```python
from build123d import *

# Parameters (mm, degrees)
SKETCH1_R           = 5
SKETCH1_W           = 15
SKETCH1_H           = 110
BOSS_EXTRUDE1_DEPTH = 10
SKETCH1_3_W         = 15
SKETCH1_3_H         = 110
BOSS_EXTRUDE2_DEPTH = 20
SKETCH2_W           = 10
SKETCH2_H           = 30
CUT_EXTRUDE1_DEPTH  = 20


with BuildPart() as part:
    # Sketch1 → Boss-Extrude1 (new body)
    with BuildSketch(Plane.XY):
        with BuildLine():
            Line((70.181538652, 27.177394162), (-59.818461348, 27.177394162))
            ThreePointArc((-59.818461348, 27.177394162), (-114.818461348, -27.822605838), (-59.818461348, -82.822605838))
            Line((-59.818461348, -82.822605838), (70.181538652, -82.822605838))
            Line((70.181538652, -82.822605838), (70.181538652, 27.177394162))
        make_face()
        with Locations((-59.818461348, -27.822605838)):
            Circle(SKETCH1_R, mode=Mode.SUBTRACT)
        with Locations((77.681538652, -27.822605838)):
            Rectangle(SKETCH1_W, SKETCH1_H)
    extrude(amount=-BOSS_EXTRUDE1_DEPTH)

    # Sketch1_3 → Boss-Extrude2 (add)
    with BuildSketch(Plane.XY):
        with Locations((77.681538652, -27.822605838)):
            Rectangle(SKETCH1_3_W, SKETCH1_3_H)
    extrude(amount=BOSS_EXTRUDE2_DEPTH)

    # Sketch2 → Cut-Extrude1 (cut)
    with BuildSketch(Plane(origin=(85.181538652, 0, 0), x_dir=(0, 0, -1), z_dir=(1, 0, 0))):
        with Locations((-5, -27.822605838)):
            Rectangle(SKETCH2_W, SKETCH2_H)
    extrude(amount=-CUT_EXTRUDE1_DEPTH, mode=Mode.SUBTRACT)


solid = part.part
```
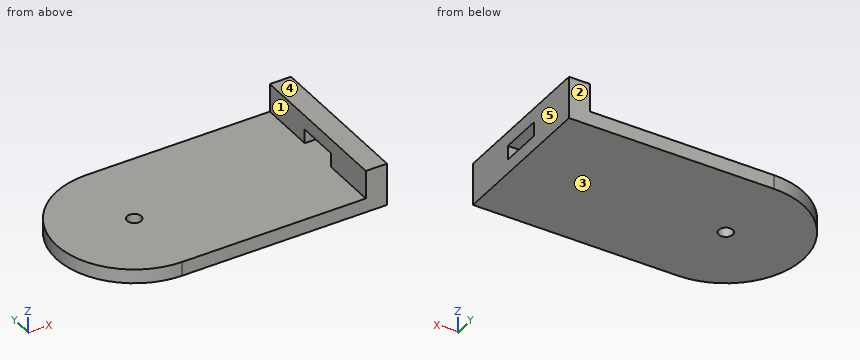
CAD build for the part. Positions are in the model's coordinates, mm. Face numbers are marked on the shaded views. A direction names the side the tool comes from. Round coordinates to 2 decimals unless told otherwise and drop trailing zeros. Order: outer loops, then holes, each group sorted by start corner. A loop starts at its lowest first (then second) coordinate and runs counter-clockwise, first axis right, second up.
Q1. Slice it at C-C (z = -7.25). Write the cut outline in (x, y), and give its area (3 significant figures).
Q2. Slice it at D-D (y = -46.5). Write the cut outline in (x, z).
Q3. Drop flat-ended pins along their axis: pin 1 (2 mm diameter, centred on x = -90, z = 2.5, fed in from -Y); pin 2 (12 mm diameter, centred on x = 43, y = -13.5, fed in from +Z); pin 3 (10 mm diameter, centred on y = -41.5, z = 12.5, fed in from -X); pin 4 (16 mm diameter, centred on y = -11.5, z = 7.5, fed in from -X). Give the stop position or say it passes through.
Q4. Which spindle directions (+Z, -Z, +X, -X, +Y, -Y) get a long thin tool onto all of the face, cutting with end or side? Do the marked faces 1 and 2. Say none if no direction does.
Q5. Two-plate mould, pull along Z, no slides. Class the marked faces 3, 4 and 5: pulls with the +Z half, pulls with the -Z half, needs draft (parallel to the pull), parting line crosses it, or undercut.
Q6. Slice it at A-A (z = 2.5). Write the cut outline in (x, y), and give its area (3 significant figures).
Q7. Wall check: L1, parallel to Z at x = -66.5, y = -25.5; L2, parallel to X at y = -22.5, z = 11.25; L3, parallel to X at y = 15, z = -6. Give the ranges that are in metal, low to high.
Q8. Slice it at B-B (y = -17.5). Write the cut outline in (x, z).
Results below:
1. outline: (-59.82, -82.82) - (85.18, -82.82) - (85.18, 27.18) - (-59.82, 27.18) arc R55 ccw to start; hole circle Ø10 at (-59.82, -27.82)
1. area: 20,600 mm2
2. outline: (-111.55, -10) - (85.18, -10) - (85.18, 20) - (70.18, 20) - (70.18, 0) - (-111.55, 0) - close
3. pin 1: passes through
3. pin 2: stops at z = 0
3. pin 3: stops at x = 70.18
3. pin 4: stops at x = -113.13
4. face 1: +Z, -X, +Y, -Y
4. face 2: +Z, -Z, +X, -X, +Y
5. face 3: pulls with the -Z half
5. face 4: pulls with the +Z half
5. face 5: needs draft
6. outline: (70.18, -82.82) - (85.18, -82.82) - (85.18, -42.82) - (70.18, -42.82) - close; (70.18, -12.82) - (85.18, -12.82) - (85.18, 27.18) - (70.18, 27.18) - close
6. area: 1,200 mm2
7. L1: z = -10 to 0
7. L2: x = 70.18 to 85.18
7. L3: x = -94.33 to 85.18
8. outline: (-113.84, -10) - (85.18, -10) - (85.18, 0) - (-113.84, 0) - close; (70.18, 10) - (85.18, 10) - (85.18, 20) - (70.18, 20) - close
